Geometry: final body of the model. Coordinates: model frame, mm. Face numbers are marked on the shaded views. Give positions to 0.01 mm unless a question says otherwise; leave off trailing zeros. Order: outer loops, then holes, each group sorted by start corner. A loop starts at its lowest first (then second) coordinate and runs counter-clockwise, first axis right, second up. Notation, with made-up numbers: (89.25, 23) - (97.25, 23) arc R32 cw to (97.25, 62) - close; hole circle Ø1 at (31, 1). An arc over 180 degrees is marked (long way). Put each result on its own line as item: value. Start each with the question number.
1. Section A-A on x = 0. Return the cut outline in (y, z), plus the area to 4 significant figures.
2. Mould query, pull axis Y, two halves, no side actions, for the marked faces 1 and 2. Classes: pulls with the +Y half, pulls with the -Y half, needs draft (parallel to the pull), parting line crosses it, or undercut.
3. First-contact query: P1, Ø8.5, axis at x = 5, y = 4, coming from the -Z side; P2, Ø1.6, axis at y = 23, z = 2.5, coming from the -X side; P3, Ø0.9, axis at y = 21.5, z = 2, coming from the -X side. Flat tips, straight axial feed; report the tip coordinate or a pass-through.
4. Section B-B on y = -5. Return the cut outline in (x, z), plus the area to 3 significant figures.
5. Ray query, line 1 along Y through (x, z) = (21.5, 2.55); line 2 along Y through (x, z) = (-5, 1.45); line 3 along X through (y, z) = (-13, 1.25). Return the intervals inside material, ascending. Write a range as from..to.
6. Section D-D on z = 2.05. Count the separate pieces of the cut face and the enclosed holes in it, plus the area to 3 significant figures.
7. Section C-C on y = 5. Return the cut outline in (x, z), plus the area to 3 significant figures.
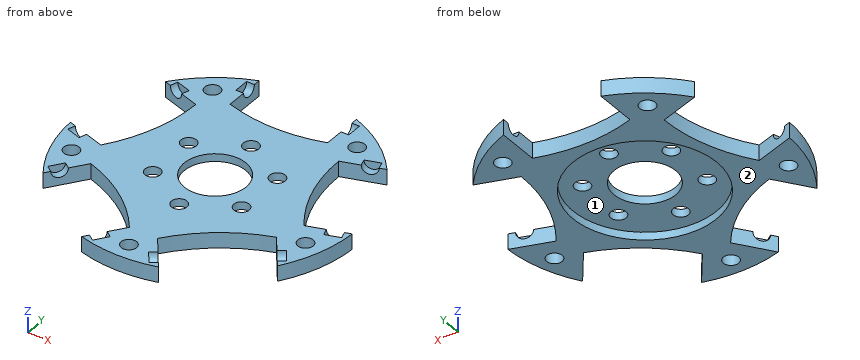
from build123d import *

# Parameters (mm, degrees)
BOSS_EXTRUDE1_DEPTH = 3
SKETCH2_R           = 1.5
SKETCH2_R_2         = 6
CUT_EXTRUDE1_DEPTH  = 3
SKETCH5_W           = 22
SKETCH5_H           = 1.5
CIRPATTERN1_COUNT   = 5
SKETCH6_R           = 14
CUT_EXTRUDE2_DEPTH  = 1.5


with BuildPart() as part:
    # Sketch1 → Boss-Extrude1 (new body)
    with BuildSketch(Plane.XY):
        with BuildLine():
            Line((-9.5, 25.806975801), (-9.5, 17.737494192))
            ThreePointArc((-9.5, 17.737494192), (0, 16.25), (9.5, 17.737494192))
            Line((9.5, 17.737494192), (9.5, 25.806975801))
            ThreePointArc((9.5, 25.806975801), (16.164094438, 22.247967345), (21.608231055, 17.009831001))
            Line((21.608231055, 17.009831001), (13.933697987, 14.516224048))
            ThreePointArc((13.933697987, 14.516224048), (15.45466839, 5.021526159), (19.805020881, -3.553849762))
            Line((19.805020881, -3.553849762), (27.479553948, -1.060242809))
            ThreePointArc((27.479553948, -1.060242809), (26.154054198, -8.497967345), (22.854621229, -15.2943221))
            Line((22.854621229, -15.2943221), (18.111498945, -8.765974342))
            ThreePointArc((18.111498945, -8.765974342), (9.55151035, -13.146526159), (2.740176052, -19.933894136))
            Line((2.740176052, -19.933894136), (7.483298336, -26.462241893))
            ThreePointArc((7.483298336, -26.462241893), (0, -27.5), (-7.483298336, -26.462241893))
            Line((-7.483298336, -26.462241893), (-2.740176052, -19.933894136))
            ThreePointArc((-2.740176052, -19.933894136), (-9.55151035, -13.146526159), (-18.111498945, -8.765974342))
            Line((-18.111498945, -8.765974342), (-22.854621229, -15.2943221))
            ThreePointArc((-22.854621229, -15.2943221), (-26.154054198, -8.497967345), (-27.479553948, -1.060242809))
            Line((-27.479553948, -1.060242809), (-19.805020881, -3.553849762))
            ThreePointArc((-19.805020881, -3.553849762), (-15.45466839, 5.021526159), (-13.933697987, 14.516224048))
            Line((-13.933697987, 14.516224048), (-21.608231055, 17.009831001))
            ThreePointArc((-21.608231055, 17.009831001), (-16.164094438, 22.247967345), (-9.5, 25.806975801))
        make_face()
    extrude(amount=BOSS_EXTRUDE1_DEPTH)

    # Sketch2 → Cut-Extrude1 (cut)
    with BuildSketch(Plane.XY.offset(3)):
        with Locations((0, 10)):
            Circle(SKETCH2_R)
        with Locations((-8.660254038, 5)):
            Circle(SKETCH2_R)
        with Locations((-8.660254038, -5)):
            Circle(SKETCH2_R)
        with Locations((0, -10)):
            Circle(SKETCH2_R)
        with Locations((8.660254038, -5)):
            Circle(SKETCH2_R)
        with Locations((8.660254038, 5)):
            Circle(SKETCH2_R)
        Circle(SKETCH2_R_2)
        with Locations((14.106846055, 19.416407865)):
            Circle(SKETCH2_R)
        with Locations((22.825356391, -7.416407865)):
            Circle(SKETCH2_R)
        with Locations((0, -24)):
            Circle(SKETCH2_R)
        with Locations((-22.825356391, -7.416407865)):
            Circle(SKETCH2_R)
        with Locations((-14.106846055, 19.416407865)):
            Circle(SKETCH2_R)
    extrude(amount=-CUT_EXTRUDE1_DEPTH, mode=Mode.SUBTRACT)

    # Sketch5 → Cut-Revolve1 (revolve, cut)
    with BuildSketch(Plane.XY.offset(3)):
        with Locations((0, 23.75)):
            Rectangle(SKETCH5_W, SKETCH5_H)
    cut_revolve1 = revolve(axis=Axis((-11, 23, 3), (1, 0, 0)), mode=Mode.SUBTRACT)

    # CirPattern1: Cut-Revolve1 ×5 about axis
    cirpattern1_axis = Axis((0, 0, 0), (0, 0, 1))
    for i in range(1, CIRPATTERN1_COUNT):
        add(cut_revolve1.rotate(cirpattern1_axis, i * 360 / CIRPATTERN1_COUNT), mode=Mode.SUBTRACT)

    # Sketch6 → Cut-Extrude2 (cut)
    with BuildSketch(Plane(origin=(0, 0, 0), x_dir=(-1, 0, 0), z_dir=(0, 0, -1))):
        Circle(SKETCH6_R)
    extrude(amount=-CUT_EXTRUDE2_DEPTH, mode=Mode.SUBTRACT)


solid = part.part
Resolved:
1. outline: (-27.5, 0) - (-25.5, 0) - (-25.5, 3) - (-27.5, 3) - close; (-22.5, 0) - (-14, 0) - (-14, 1.5) - (-11.5, 1.5) - (-11.5, 3) - (-22.5, 3) - close; (-8.5, 1.5) - (-6, 1.5) - (-6, 3) - (-8.5, 3) - close; (6, 1.5) - (8.5, 1.5) - (8.5, 3) - (6, 3) - close; (11.5, 1.5) - (14, 1.5) - (14, 0) - (16.25, 0) - (16.25, 3) - (11.5, 3) - close
1. area: 53.25 mm^2
2. face 1: undercut
2. face 2: needs draft
3. P1: z = 1.5
3. P2: x = -16.23
3. P3: x = -17.7
4. outline: (-27.04, 0) - (-13.08, 0) - (-13.08, 1.5) - (-10.16, 1.5) - (-10.16, 3) - (-27.04, 3) - close; (-7.16, 1.5) - (-3.32, 1.5) - (-3.32, 3) - (-7.16, 3) - close; (3.32, 1.5) - (7.16, 1.5) - (7.16, 3) - (3.32, 3) - close; (10.16, 1.5) - (13.08, 1.5) - (13.08, 0) - (27.04, 0) - (27.04, 3) - (10.16, 3) - close
4. area: 104 mm^2
5. line 1: -11.04..-8.12, -6.71..-3, 16.97..17.15
5. line 2: -27.04..-23.04, -17.19..-13.08, 13.08..16.65
5. line 3: -24.23..-21.19, -9.75..-5.2, 5.2..9.75, 21.19..24.23
6. separate pieces: 1
6. enclosed holes: 12
6. area: 1,180 mm^2
7. outline: (-15.46, 0) - (-13.08, 0) - (-13.08, 1.5) - (-10.16, 1.5) - (-10.16, 3) - (-15.46, 3) - close; (-7.16, 1.5) - (-3.32, 1.5) - (-3.32, 3) - (-7.16, 3) - close; (3.32, 1.5) - (7.16, 1.5) - (7.16, 3) - (3.32, 3) - close; (10.16, 1.5) - (13.08, 1.5) - (13.08, 0) - (15.46, 0) - (15.46, 3) - (10.16, 3) - close
7. area: 34.6 mm^2
